```python
from build123d import *

# Parameters (mm, degrees)
BOSS_EXTRUDE1_DEPTH = 3.175


with BuildPart() as part:
    # Sketch1 → Boss-Extrude1 (new body)
    with BuildSketch(Plane(origin=(0, 0, 0), x_dir=(1, 0, 0), z_dir=(0, 1, 0))):
        Polygon((-27.49630657, 15.875), (-25.296602045, 17.145), (-24.016404155, 14.927632211), (-20.716847366, 16.832632211), (-21.997045256, 19.05), (-18.697488468, 20.955), (-17.427488468, 18.755295474), (-14.127931679, 20.660295474), (-15.397931679, 22.86), (-12.098374891, 24.765), (-10.828374891, 22.565295474), (-7.528818102, 24.470295474), (-8.798818102, 26.67), (-5.499261314, 28.575), (-4.219063424, 26.357632211), (-0.919506636, 28.262632211), (-2.199704526, 30.48), (0, 31.75), (2.199704526, 30.48), (0.919506636, 28.262632211), (4.219063424, 26.357632211), (5.499261314, 28.575), (8.798818102, 26.67), (7.528818102, 24.470295474), (10.828374891, 22.565295474), (12.098374891, 24.765), (15.397931679, 22.86), (14.127931679, 20.660295474), (17.427488468, 18.755295474), (18.697488468, 20.955), (21.997045256, 19.05), (20.716847366, 16.832632211), (24.016404155, 14.927632211), (25.296602045, 17.145), (27.49630657, 15.875), (27.49630657, 13.335), (24.935910791, 13.335), (24.935910791, 9.525), (27.49630657, 9.525), (27.49630657, 5.715), (24.95630657, 5.715), (24.95630657, 1.905), (27.49630657, 1.905), (27.49630657, -1.905), (24.95630657, -1.905), (24.95630657, -5.715), (27.49630657, -5.715), (27.49630657, -9.525), (24.935910791, -9.525), (24.935910791, -13.335), (27.49630657, -13.335), (27.49630657, -15.875), (25.296602045, -17.145), (24.016404155, -14.927632211), (20.716847366, -16.832632211), (21.997045256, -19.05), (18.697488468, -20.955), (17.427488468, -18.755295474), (14.127931679, -20.660295474), (15.397931679, -22.86), (12.098374891, -24.765), (10.828374891, -22.565295474), (7.528818102, -24.470295474), (8.798818102, -26.67), (5.499261314, -28.575), (4.219063424, -26.357632211), (0.919506636, -28.262632211), (2.199704526, -30.48), (0, -31.75), (-2.199704526, -30.48), (-0.919506636, -28.262632211), (-4.219063424, -26.357632211), (-5.499261314, -28.575), (-8.798818102, -26.67), (-7.528818102, -24.470295474), (-10.828374891, -22.565295474), (-12.098374891, -24.765), (-15.397931679, -22.86), (-14.127931679, -20.660295474), (-17.427488468, -18.755295474), (-18.697488468, -20.955), (-21.997045256, -19.05), (-20.716847366, -16.832632211), (-24.016404155, -14.927632211), (-25.296602045, -17.145), (-27.49630657, -15.875), (-27.49630657, -13.335), (-24.935910791, -13.335), (-24.935910791, -9.525), (-27.49630657, -9.525), (-27.49630657, -5.715), (-24.95630657, -5.715), (-24.95630657, -1.905), (-27.49630657, -1.905), (-27.49630657, 1.905), (-24.95630657, 1.905), (-24.95630657, 5.715), (-27.49630657, 5.715), (-27.49630657, 9.525), (-24.935910791, 9.525), (-24.935910791, 13.335), (-27.49630657, 13.335), align=None)
        Polygon((21.883093223, 12.895356956), (-0.226160103, 25.398993122), (-22.109253326, 12.503636166), (-21.883093223, -12.895356956), (0.226160103, -25.398993122), (22.109253326, -12.503636166), align=None, mode=Mode.SUBTRACT)
    extrude(amount=-BOSS_EXTRUDE1_DEPTH)


solid = part.part
```
Could you check a few things on this model? Use its own coordinates, in mm. A direction names the side the tool comes from. Round coordinates to 2 decimals unless told otherwise and drop trailing zeros. Write each loop counter-clockwise with the first axis right and the second up, starting at its lowest first coordinate (ties: lowest second). Pieces come first, ordered by that corner, then holes.
(1) Which directions (+Z, -Z, +X, -X, +Y, -Y) give clear straight access to the entire face, cutting with the end or side of a thin tool? Please do faces 1 (the face through (-22.344, -1.565, 15.893)), 2 (the face through (26, -2, 1.905)), 3 (the face through (-26, -2, 5.715)).
Findings below:
face 1: +Y, -Y
face 2: +X, +Y, -Y
face 3: -X, +Y, -Y
(2) Suppose I cut it at A-A on z = -27.5. Write out the boundary of the cut face in (x, y) (3 decimals), and give its area (3 significant figures).
Findings below:
outline: (-7.361, -3.175) - (-4.879, -3.175) - (-4.879, 0) - (-7.361, 0) - close; (-2.24, -3.175) - (2.24, -3.175) - (2.24, 0) - (-2.24, 0) - close; (4.879, -3.175) - (7.361, -3.175) - (7.361, 0) - (4.879, 0) - close
area: 30.0 mm2
(3) If I drill on probe 1 along Z at (x, y) = (-8.5, -2.8); probe 2 along X at (y, z) = (-2.3, -26.5); probe 3 along Z at (x, y) = (-14.5, -0.3), over which ranges is the centre line in solid material (lowest first)?
Findings below:
probe 1: z = -26.84 to -26.15, -23.91 to -20.52, 20.46 to 23.91, 26.15 to 26.84
probe 2: x = -8.7 to -4.3, -3.97 to 3.97, 4.3 to 8.7
probe 3: z = -23.38 to -21.3, -20.45 to -16.99, 17.07 to 20.45, 21.3 to 23.38
(4) Suppose I cut it at B-B on x = -3. Write out the boundary of the cut face in (y, z) (3 decimals), and give its area (3 significant figures).
Findings below:
outline: (-3.175, -27.061) - (0, -27.061) - (0, -23.764) - (-3.175, -23.764) - close; (-3.175, 23.574) - (0, 23.574) - (0, 27.061) - (-3.175, 27.061) - close
area: 21.5 mm2
(5) Thinking about a two-plate mould opening in X: for faces 4 (the face through (-8, 0, 21)), 5 (the face through (9.16, -1.57, -23.53)), 6 (the face through (26.38, -1.57, -16.52)), which applies, +X half, -X half, draft (parallel to the pull), parting line (faces both ways), or undercut?
Findings below:
face 4: draft
face 5: undercut
face 6: +X half
(6) For pin 1 (0.8 mm diameter, centred on x = -25.5, y = -2, fed in from -Z) (3 decimals); pin 2 (1.3 mm diameter, centred on x = -26.5, y = -1.5, fed in from +Z); pin 3 (1 mm diameter, centred on y = -1.5, z = 3.5, fed in from +X), each with a flat end and sliding along its axis, tell me the tip position at first contact or that it passes through.
Findings below:
pin 1: stops at z = -17.145
pin 2: stops at z = 16.83
pin 3: stops at x = 24.96
(7) Suppose I cut it at C-C on z = 11. Write out the boundary of the cut face in (x, y) (3 decimals), and give its area (3 significant figures).
Findings below:
outline: (-24.936, -3.175) - (-21.9, -3.175) - (-21.9, 0) - (-24.936, 0) - close; (22.096, -3.175) - (24.936, -3.175) - (24.936, 0) - (22.096, 0) - close
area: 18.7 mm2
